Verification items for the finished model (mm, model axes). Give positions to 0.01 mm unless a question says otherwise; leave off trailing zeros. Write each loop counter-clockwise with the first axis right and the second up, starting at its lowest first coordinate (ties: lowest second). Pieces come first, ordered by that corner, then holes. Notation, with made-up numbers: (-22.75, -34.5) -> (5.25, -34.5) arc R21 cw to (5.25, -6.5) -> close; hole circle Ø6 at (38.5, 13). An arc over 180 degrees is marked (long way). Use one line per item in the form item = value. Start each with the question number.
(1) Depth check by flat-ended pin: pin 1 Ø1 at (y, z) = (-34, -1) entering from -X. Enter the tip coordinate at first touch or a pass-through.
(2) Section check B-B, the plane y = -35. Record the cut outline in (x, z).
(3) Release check for a two-part mould opening along X. For faces 1 (the face through (-0.56, -37.54, -1.48)), 2 (the face through (0, -13, -1)), 3 (the face through (-7.5, -37.9, -1.5)) record: pulls with the +X half, pulls with the -X half, needs draft (parallel to the pull), parting line crosses it, or undercut.
(4) Section check D-D, the plane x = -4.5. Record the cut outline in (y, z).
(5) Section check A-A, the plane x = 1. Record the cut outline in (y, z), plus the area to 3 significant figures.
(6) Section check C-C, the plane z = -1.6. Record the cut outline in (x, y).
(7) Scan lines: L1, parallel to Y at x = 0, z = -2.3; L2, parallel to Y at x = -2.25, z = -0.1; L3, parallel to X at y = -18.5, z = -1.55. Record each from-to range of solid material in increasing order.
from build123d import *

# Parameters (mm, degrees)
SKETCH1_R          = 2.6
BASE_FLANGE1_DEPTH = 3
FILLET1_R          = 7


# Sheet-metal steps are written as plain solids
with BuildPart() as part:
    # Sketch1 → Base-Flange1 (new body)
    with BuildSketch(Plane.XY):
        with BuildLine():
            Line((-9.5, -13), (-9.5, -33))
            ThreePointArc((-9.5, -33), (-7.449747468, -37.949747468), (-2.5, -40))
            Line((-2.5, -40), (2.5, -40))
            ThreePointArc((2.5, -40), (7.449747468, -37.949747468), (9.5, -33))
            Line((9.5, -33), (9.5, -13))
            Line((9.5, -13), (-9.5, -13))
        make_face()
        with Locations((0, -35)):
            Circle(SKETCH1_R, mode=Mode.SUBTRACT)
        with Locations((0, -20)):
            Circle(SKETCH1_R, mode=Mode.SUBTRACT)
    extrude(amount=-BASE_FLANGE1_DEPTH)

    # Fillet1
    fillet1_edges = [part.edges().sort_by_distance(p)[0] for p in [
        (9.5, -13, -1.5),
        (-9.5, -13, -1.5),
    ]]
    fillet(fillet1_edges, radius=FILLET1_R)


solid = part.part
Completed:
q1.pin_1 = -9.48
q2.outline = (-9.21, -3) -> (-2.6, -3) -> (-2.6, 0) -> (-9.21, 0) -> close; (2.6, -3) -> (9.21, -3) -> (9.21, 0) -> (2.6, 0) -> close
q3.face_1 = undercut
q3.face_2 = needs draft
q3.face_3 = pulls with the -X half
q4.outline = (-39.71, -3) -> (-13.29, -3) -> (-13.29, 0) -> (-39.71, 0) -> close
q5.outline = (-40, -3) -> (-37.4, -3) -> (-37.4, 0) -> (-40, 0) -> close; (-32.6, -3) -> (-22.4, -3) -> (-22.4, 0) -> (-32.6, 0) -> close; (-17.6, -3) -> (-13, -3) -> (-13, 0) -> (-17.6, 0) -> close
q5.area = 52.2 mm²
q6.outline = (-9.5, -33) arc R7 ccw to (-2.5, -40) -> (2.5, -40) arc R7 ccw to (9.5, -33) -> (9.5, -20) arc R7 ccw to (2.5, -13) -> (-2.5, -13) arc R7 ccw to (-9.5, -20) -> close; hole circle Ø5.2 at (0, -35); hole circle Ø5.2 at (0, -20)
q7.L1 = -40 to -37.6, -32.4 to -22.6, -17.4 to -13
q7.L2 = -40 to -36.3, -33.7 to -21.3, -18.7 to -13
q7.L3 = -9.34 to -2.12, 2.12 to 9.34
